from build123d import *

# Parameters (mm, degrees)
F0_R     = 32
F0_R_2   = 12
F1_DEPTH = 7
F3_D     = 2.5
F4_DEPTH = 2.5
F5_R     = 0.75
F6_DEPTH = 25
F7_W     = 18.952996
F7_H     = 20.40381
F8_DEPTH = 25


with BuildPart() as f1:
    # F0 (on Top) → F1 (new body)
    with BuildSketch(Plane.XY):
        Circle(F0_R)
        Circle(F0_R_2, mode=Mode.SUBTRACT)
    extrude(amount=F1_DEPTH)

    # F3 (through all)
    with Locations(Plane.XY.offset(7)):
        with Locations((-15.202796, 15.202796), (15.202796, 15.202796), (15.202796, -15.202796), (-15.202796, -15.202796)):
            Hole(F3_D / 2)

    # F2 (on face) → F4 (cut)
    with BuildSketch(Plane.XY.offset(7)):
        Polygon((-12.158075, 15.817457), (-14.212748, 18.146932), (-17.257468, 17.532271), (-18.247517, 14.588135), (-16.192844, 12.25866), (-13.148123, 12.873321), align=None)
        Polygon((12.25866, 16.192844), (12.873321, 13.148123), (15.817457, 12.158075), (18.146932, 14.212748), (17.532271, 17.257468), (14.588135, 18.247517), align=None)
        Polygon((16.192844, -12.25866), (13.148123, -12.873321), (12.158075, -15.817457), (14.212748, -18.146932), (17.257468, -17.532271), (18.247517, -14.588135), align=None)
        Polygon((-12.25866, -16.192844), (-12.873321, -13.148123), (-15.817457, -12.158075), (-18.146932, -14.212748), (-17.532271, -17.257468), (-14.588135, -18.247517), align=None)
    extrude(amount=-F4_DEPTH, mode=Mode.SUBTRACT)

    # F5 (on Top) → F6 (cut)
    with BuildSketch(Plane.XY):
        with Locations((-25, 0)):
            Circle(F5_R)
        with Locations((0, -25)):
            Circle(F5_R)
        with Locations((25, 0)):
            Circle(F5_R)
        with Locations((0, 25)):
            Circle(F5_R)
    extrude(amount=F6_DEPTH, mode=Mode.SUBTRACT)

    # F7 (on Top) → F8 (cut)
    with BuildSketch(Plane.XY):
        with Locations((0, -32.00157)):
            Rectangle(F7_W, F7_H)
    extrude(amount=F8_DEPTH, mode=Mode.SUBTRACT)


solid = f1.part
The listing builds one solid part. Answer for the finished solid, in the listing's coordinates (mm). A direction names the side the tool comes from. Give positions to 0.01 mm unless a question says otherwise; leave off trailing zeros. Write each loop counter-clockwise with the first axis right and the second up, starting at its lowest first coordinate (ties: lowest second). Pieces come first, ordered by that corner, then holes.
Item 1: Section B-B, the plane x = 0 is taken. Write down the section's boundary in (y, z), plus the area to 3 significant figures.
Item 2: Section D-D, the plane x = 7.5 is taken. Write down the section's boundary in (y, z).
Item 3: Section C-C, the plane z = 5.5 is taken. Count the separate pieces of the cut face and the enclosed holes in it, plus the area to 3 significant figures.
Item 4: Find the intervals of material crossed by line 1 along X through (y, z) = (-16, 1.75); line 2 along X through (y, z) = (25, 3.5); line 3 along Y through (x, z) = (9, 5), in increasing order.
Item 5: Which of the six approach directions +Z, -Z, +X, -X, +Y, -Y give full straight-line access (tool end or side, diameter ignored) to faces 1 (the flat face through (-15, 17, 4.5)), 2 (the flat face through (-9.476, -26, 3)), 3 (the cylindrical face through (-14.932, -16.423, 2.219))?
Item 6: Section A-A, the plane y = 0 is taken. Write down the section's boundary in (x, z).
Item 7: Flat-ended cylindrical pins translate along their axes: P1, Ø4, axis at x = -15.2, y = 15.2, coming from the +Z side; P2, Ø2, axis at x = 2.5, z = 3.5, coming from the -Y side; P3, Ø4, axis at y = 23.5, z = 1.5, coming from the +X side. Find the tip coordinate at first contact, or state that the pin passes through.
Completed:
1. outline: (-21.8, 0) - (-12, 0) - (-12, 7) - (-21.8, 7) - close; (12, 0) - (24.25, 0) - (24.25, 7) - (12, 7) - close; (25.75, 0) - (32, 0) - (32, 7) - (25.75, 7) - close
1. area: 198 mm2
2. outline: (-21.8, 0) - (-9.37, 0) - (-9.37, 7) - (-21.8, 7) - close; (9.37, 0) - (31.11, 0) - (31.11, 7) - (9.37, 7) - close
3. separate pieces: 1
3. enclosed holes: 8
3. area: 2,470 mm2
4. line 1: x = -27.71 to -16.17, -14.24 to 14.24, 16.17 to 27.71
4. line 2: x = -19.97 to -0.75, 0.75 to 19.97
4. line 3: y = -21.8 to -7.94, 7.94 to 30.71
5. face 1: +Z
5. face 2: +Z, -Z, -Y
5. face 3: +Z, -Z
6. outline: (-32, 0) - (-25.75, 0) - (-25.75, 7) - (-32, 7) - close; (-24.25, 0) - (-12, 0) - (-12, 7) - (-24.25, 7) - close; (12, 0) - (24.25, 0) - (24.25, 7) - (12, 7) - close; (25.75, 0) - (32, 0) - (32, 7) - (25.75, 7) - close
7. P1: stops at z = 4.5
7. P2: stops at y = -21.8
7. P3: stops at x = 23.7
